Could you check a few things on this model? Use its own coordinates, in mm. Face numbers are marked on the shaded views. A direction names the side the tool comes from. Give positions to 0.01 mm unless a question says otherwise; leave off trailing zeros. Order: outer loops, then holes, each group sorted by start corner. A loop starts at its lowest first (then second) coordinate and runs counter-clockwise, first axis right, second up. Notation, with made-up numbers: (83.5, -1.75) -> (137.5, -1.75) arc R31 ccw to (137.5, 23.25) -> close; hole circle Ø2 at (62, 53.5). An arc over 180 degrees is marked (long way). One line per item, written item: value.
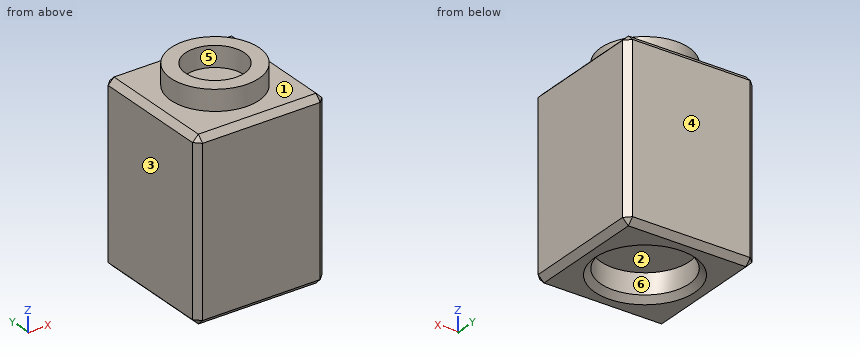
```python
from build123d import *

# Parameters (mm, degrees)
F2_W     = 44
F2_H     = 44
F2_R     = 15
F2_R_2   = 10
F3_DEPTH = 60
F4_R     = 15
F4_R_2   = 10
F5_DEPTH = 7
F6_DEPTH = 9
F8_SIZE  = 2


with BuildPart() as f3:
    # F2 (on Top) → F3 (new body)
    with BuildSketch(Plane.XY):
        Rectangle(F2_W, F2_H)
        Circle(F2_R, mode=Mode.SUBTRACT)
        Circle(F2_R)
        Circle(F2_R_2, mode=Mode.SUBTRACT)
        Circle(F2_R_2)
    extrude(amount=F3_DEPTH)

    # F4 (on face) → F5 (join)
    with BuildSketch(Plane.XY.offset(60)):
        Circle(F4_R)
        Circle(F4_R_2, mode=Mode.SUBTRACT)
    extrude(amount=F5_DEPTH)

    # F2 (on Top) → F6 (cut)
    with BuildSketch(Plane.XY):
        Circle(F2_R)
        Circle(F2_R_2, mode=Mode.SUBTRACT)
        Circle(F2_R_2)
    extrude(amount=F6_DEPTH, mode=Mode.SUBTRACT)

    # F8
    f8_edges = [f3.edges().sort_by_distance(p)[0] for p in [
        (0, -22, 0),
        (22, 0, 0),
        (-22, 0, 0),
        (0, 22, 0),
        (-22, -22, 30),
        (-22, 22, 30),
        (22, 22, 30),
        (22, -22, 30),
        (22, 0, 60),
        (0, -22, 60),
        (-22, 0, 60),
        (0, 22, 60),
        (-15, 0, 0),
    ]]
    chamfer(f8_edges, length=F8_SIZE)


solid = f3.part
```
1) We'd pull the mould along X, two halves only. Please class the marked faces 1, 2 and 3: +X half, -X half, draft (parallel to the pull), parting line (faces both ways), or undercut.
Answer below:
face 1: draft
face 2: undercut
face 3: -X half
2) For P1, Ø18, axis at x = 0, y = 0, coming from the +Z side, with a flat end and sliding along its axis, tell me the tip position at first contact or that it passes through.
Answer below:
P1: stops at z = 60
3) If I drill on line 1 along Y through (x, z) = (0, 6); line 2 along Y through (x, z) = (0, 64.75); line 3 along Z through (x, y) = (19.5, -19), over which ranges is the centre line in solid material (lowest first)?
Answer below:
line 1: y = -22 to -15, 15 to 22
line 2: y = -15 to -10, 10 to 15
line 3: z = 0 to 60
4) Suppose I cut it at A-A, the plane y = 0. Write out the boundary of the cut face in (x, z).
Answer below:
outline: (-22, 2) -> (-20, 0) -> (-17, 0) -> (-15, 2) -> (-15, 9) -> (15, 9) -> (15, 2) -> (17, 0) -> (20, 0) -> (22, 2) -> (22, 58) -> (20, 60) -> (15, 60) -> (15, 67) -> (10, 67) -> (10, 60) -> (-10, 60) -> (-10, 67) -> (-15, 67) -> (-15, 60) -> (-20, 60) -> (-22, 58) -> close
5) For the marked faces 4, 5 and 6, which set-ups out of +Z, -Z, +X, -X, +Y, -Y let a thin tool reach every point of the face, with its end or its side?
Answer below:
face 4: +Z, -Z, +X, -X, +Y
face 5: +Z
face 6: -Z
